Check sheet for the modelled part. Datum: model origin and axes. Units: mm. Give positions to 0.01 mm unless a question says otherwise; leave off trailing zeros. Order: outer loops, then holes, each group sorted by start corner. A loop starts at its lowest first (then second) coordinate and runs counter-clockwise, first axis right, second up. Notation, with made-up numbers: M 60,-2 L 110,-2 A10 cw 110,8 Z; hole C 19,54 d8. An arc over 180 degrees is marked long. Return JSON: item names as keys, results as strings. Group by question number.
Autodesk Inventor part; units mm, degrees
ref_plane "YZ Plane" through (0, 0, 0) normal (1, 0, 0) x (0, 1, 0)
ref_plane "XZ Plane" through (0, 0, 0) normal (0, 1, 0) x (-1, 0, 0)
ref_plane "XY Plane" through (0, 0, 0) normal (0, 0, 1) x (1, 0, 0)
sketch "Sketch1" plane through (0, 0, 0) normal (0, 0, 1) x (1, 0, 0)
  line L0 (-100, 100) -> (100, 100)
  line L1 (100, 100) -> (100, -100)
  line L2 (100, -100) -> (-100, -100)
  line L3 (-100, -100) -> (-100, 100)
  line L4 (-100, 100) -> (100, -100) construction
  line L5 (100, 100) -> (-100, -100) construction
  point P0 (0, 0)
  dimension "d0" = 200
  dimension "d1" = 200
extrude "Plate1" add sketch "Sketch1" along normal blind 4
sketch "Sketch2" plane through (0, 0, 0) normal (0, 0, 1) x (1, 0, 0)
  circle A0 centre (0, 0) radius 45
  dimension "d3" = 90
extrude "Extrusion1" cut sketch "Sketch2" along normal blind 10
equation "\"d1\" = d0"
equation "\"d2\" = Thickness"
equation "\"BendRadius\" = Thickness"
equation "\"BendReliefWidth\" = Thickness"
equation "\"BendReliefDepth\" = 0.5 * Thickness"
equation "\"CornerReliefSize\" = 4 * Thickness"
equation "\"MinimumRemnant\" = 2 * Thickness"
equation "\"TransitionRadius\" = BendRadius"
equation "\"JacobiRadiusSize\" = BendRadius"
equation "\"GapSize\" = Thickness"
equation "\"Конус_Угол_продольный\" = 52.4deg"
equation "\"Конус_Угол_поперечный\" = 52deg"
equation "\"Конус_Дно_сторона\" = 200"
equation "\"Конус_ширина_по_оси\" = 1700"
properties part number "MSC 011 Cone IN bottom" material "Stainless Steel"
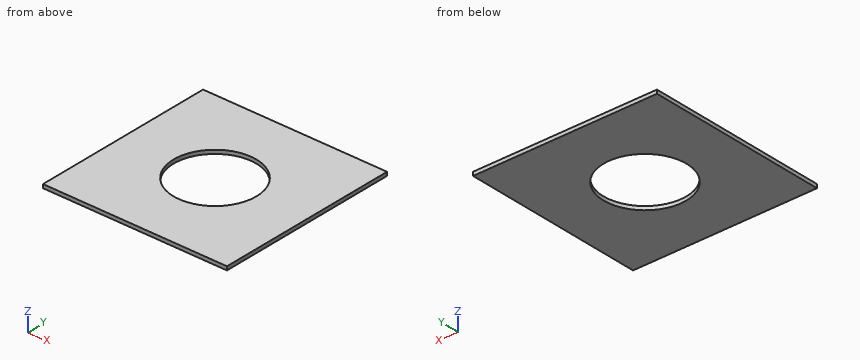
1) Material ranges on line 1 along X through (y, z) = (0, 2.15); line 2 along X through (y, z) = (31.5, 1.1), recorded low to high.
2) Sectioned sample at A-A on x = 0. Record the boundary of the cut face in (y, z).
3) Sectioned sample at C-C on z = 1.3. Record the boundary of the cut face in (x, y), then the cut area to 3 significant figures.
Reply:
{
 "1": {"line 1": "-100 to -45, 45 to 100", "line 2": "-100 to -32.14, 32.14 to 100"},
 "2": {"outline": "M -100,0 L -45,0 L -45,4 L -100,4 Z; M 45,0 L 100,0 L 100,4 L 45,4 Z"},
 "3": {"outline": "M -100,-100 L 100,-100 L 100,100 L -100,100 Z; hole C 0,0 d90", "area": "33,600 mm^2"}
}
